from build123d import *

# Parameters (mm, degrees)
F0_R     = 2.54
F1_DEPTH = 5.08


with BuildPart() as f1:
    # F0 (on Front) → F1 (new body)
    with BuildSketch(Plane.XZ):
        with BuildLine():
            ThreePointArc((-48.909848, -34.724761), (-47.497862, -32.648118), (-47.001315, -30.186494))
            ThreePointArc((-47.001315, -30.186494), (-50.705854, -24.413797), (-57.497075, -25.37659))
            ThreePointArc((-57.497075, -25.37659), (-58.29029, -34.177612), (-49.518854, -35.249571))
            Line((-49.518854, -35.249571), (-48.909848, -34.724761))
        make_face()
        with Locations((-53.351315, -30.186494)):
            Circle(F0_R, mode=Mode.SUBTRACT)
        with BuildLine():
            ThreePointArc((-57.497075, -25.37659), (-50.705854, -24.413797), (-47.001315, -30.186494))
            ThreePointArc((-47.001315, -30.186494), (-47.497862, -32.648118), (-48.909848, -34.724761))
            Line((-48.909848, -34.724761), (46.992039, 47.918384))
            ThreePointArc((46.992039, 47.918384), (38.03665, 48.583185), (38.701002, 57.538608))
            Line((38.701002, 57.538608), (-57.497075, -25.37659))
        make_face()
        with BuildLine():
            ThreePointArc((-49.518854, -35.249571), (-49.206037, -34.996814), (-48.909848, -34.724761))
            Line((-48.909848, -34.724761), (-49.518854, -35.249571))
        make_face()
        with BuildLine():
            ThreePointArc((49.196762, 52.728704), (45.492222, 58.501402), (38.701002, 57.538608))
            ThreePointArc((38.701002, 57.538608), (38.03665, 48.583185), (46.992039, 47.918384))
            ThreePointArc((46.992039, 47.918384), (48.619327, 50.082954), (49.196762, 52.728704))
        make_face()
        with Locations((42.846762, 52.728704)):
            Circle(F0_R, mode=Mode.SUBTRACT)
    extrude(amount=F1_DEPTH)


solid = f1.part
Build history of the part. All positions in model axes, mm. Give positions to 0.01 mm unless a question says otherwise; leave off trailing zeros. Write each loop counter-clockwise with the first axis right and the second up, starting at its lowest first coordinate (ties: lowest second). Pieces come first, ordered by that corner, then holes. Notation, with made-up numbers: (74, 2.5) - (95, 2.5) arc R25 cw to (95, 22.5) - close; hole circle Ø3 at (84, 69). An arc over 180 degrees is marked (long way). Use one line per item in the form item = value. Start each with the question number.
1. Probe line 1 (Z direction, x = -43, y = -1.3); line 2 (Z direction, x = 42, y = -2.7); line 3 (Z direction, x = -44, y = -4.2). List the from-to ranges inside material, lowest first. Write a range as [from, to].
2. Band-saw the part on B-B on z = 40. Write the cut outline in (x, y), plus the area to 3 significant figures.
3. Drop flat-ended pins along their axis: pin 1 Ø1.5 at (x, y) = (20, -2.5) entering from +Z; pin 2 Ø1 at (x, y) = (15.5, -2.5) entering from -Z. Give the stop position or say it passes through.
4. Band-saw the part on C-C on x = 32.5. Write the cut outline in (y, z), plus the area to 3 significant figures.
5. Band-saw the part on A-A on y = -1.3. Write the cut outline in (x, z).
Conclusion:
q1.line_1 = [-29.63, -12.88]
q1.line_2 = [43.62, 50.33], [55.12, 59.02]
q1.line_3 = [-30.49, -13.74]
q2.outline = (18.35, -5.08) - (37.8, -5.08) - (37.8, 0) - (18.35, 0) - close
q2.area = 98.8 mm²
q3.pin_1 = 42.07
q3.pin_2 = 20.35
q4.outline = (-5.08, 35.43) - (0, 35.43) - (0, 52.19) - (-5.08, 52.19) - close
q4.area = 85.2 mm²
q5.outline = (-57.5, -25.38) arc R6.35 ccw to (-49.52, -35.25) arc R6.35 ccw to (-48.91, -34.72) - (46.99, 47.92) arc R6.35 ccw to (38.7, 57.54) - close; hole circle Ø5.08 at (-53.35, -30.19); hole circle Ø5.08 at (42.85, 52.73)
